Geometry: see drawing. Coordinates: mm, zero at the bounding-box minimum. Coordinates: 2 decimals unless noted, no trailing zeros. Write each loop counter-clockwise with the first axis right and the second up, starting at its lowest first coordinate (ties: lowest second). Pieces come first, ordered by that corner, then holes. Notation, with made-up numbers: (38.25, 45) - (82.25, 45) arc R12 cw to (82.25, 53) - close; hole circle Ø7 at (5.5, -38.75). An arc over 180 degrees is marked (long way). Use CSV: the item, a comma, the result in double quotes.
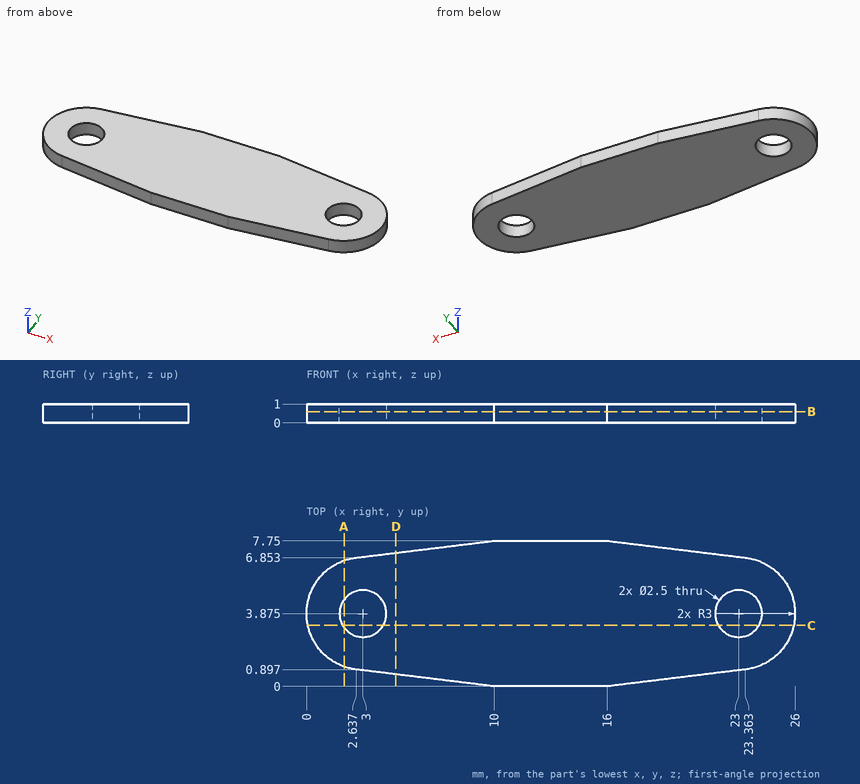
(1) Cut plane D-D on x = 4.75. Return loops of the section in (y, z).
Check values:
outline,"(0.64, 0) - (7.11, 0) - (7.11, 1) - (0.64, 1) - close"
(2) Cut plane A-A on x = 2. Return loops of the section in (y, z) (1 decimal).
Check values:
outline,"(1, 0) - (3.1, 0) - (3.1, 1) - (1, 1) - close; (4.6, 0) - (6.7, 0) - (6.7, 1) - (4.6, 1) - close"
(3) Cut plane C-C on y = 3.25. Return loops of the section in (x, z).
Check values:
outline,"(0.07, 0) - (1.92, 0) - (1.92, 1) - (0.07, 1) - close; (4.08, 0) - (21.92, 0) - (21.92, 1) - (4.08, 1) - close; (24.08, 0) - (25.93, 0) - (25.93, 1) - (24.08, 1) - close"
(4) Ray query, probe 1 along X at (y, z) = (4, 0.35); probe 2 along X at (y, z) = (5, 0.5) (1 decimal); probe 3 along Y at (x, z) = (3, 0.5) (1 decimal). Return the intervals inside material, ascending. Write a range as from..to.
Check values:
probe 1,"0..1.76, 4.24..21.76, 24.24..26"
probe 2,"0.2..2.5, 3.5..22.5, 23.5..25.8"
probe 3,"0.9..2.6, 5.1..6.9"
(5) Pin query (flat end, axial travel): pin 1 Ø3 at (x, y) = (3, 3.875) entering from -Z. Return the tip coordinate at first contact, or that it passes through.
Check values:
pin 1,"z = 0"
(6) Cut plane B-B on z = 0.6. State how many separate pieces and enclosed holes the cut face has.
Check values:
separate pieces,"1"
enclosed holes,"2"
